```python
from build123d import *

# Parameters (mm, degrees)
SKETCH1_W                                            = 50
SKETCH1_H                                            = 68
BOSS_EXTRUDE1_DEPTH                                  = 8
M3_CLEARANCE_HOLE1_D                                 = 3.4
CSK_FOR_M4_HEX_SOCKET_COUNTERSUNK_CAP_SC_D           = 4.5
CSK_FOR_M4_HEX_SOCKET_COUNTERSUNK_CAP_SC_CSINK_D     = 8.96
CSK_FOR_M4_HEX_SOCKET_COUNTERSUNK_CAP_SC_CSINK_ANGLE = 90
FILLET1_R                                            = 2
CSK_FOR_M4_HEX_SOCKET_COUNTERSUNK_CA_2_D             = 4.5
CSK_FOR_M4_HEX_SOCKET_COUNTERSUNK_CA_2_CSINK_D       = 8.96
CSK_FOR_M4_HEX_SOCKET_COUNTERSUNK_CA_2_CSINK_ANGLE   = 90


with BuildPart() as part:
    # Sketch1 → Boss-Extrude1 (new body)
    with BuildSketch(Plane(origin=(0, 0, 0), x_dir=(0, 0, -1), z_dir=(1, 0, 0))):
        Rectangle(SKETCH1_W, SKETCH1_H)
    extrude(amount=BOSS_EXTRUDE1_DEPTH)

    # M3 Clearance Hole1 (through all)
    with Locations(Plane(origin=(8, 0, 0), x_dir=(0, 0, -1), z_dir=(1, 0, 0))):
        with Locations((-10, 21), (10, 21), (10, 1), (-10, 1)):
            Hole(M3_CLEARANCE_HOLE1_D / 2)

    # CSK for M4 Hex Socket Countersunk Cap Sc (through all)
    with Locations(Plane.ZY):
        with Locations((-20, -29), (20, -29)):
            CounterSinkHole(CSK_FOR_M4_HEX_SOCKET_COUNTERSUNK_CAP_SC_D / 2, CSK_FOR_M4_HEX_SOCKET_COUNTERSUNK_CAP_SC_CSINK_D / 2, counter_sink_angle=CSK_FOR_M4_HEX_SOCKET_COUNTERSUNK_CAP_SC_CSINK_ANGLE)

    # Fillet1
    fillet1_edges = [part.edges().sort_by_distance(p)[0] for p in [
        (4, -34, -25),
        (4, -34, 25),
        (4, 34, 25),
        (4, 34, -25),
    ]]
    fillet(fillet1_edges, radius=FILLET1_R)

    # CSK for M4 Hex Socket Countersunk Ca 2 (through all)
    with Locations(Plane.ZY):
        with Locations((20, -19), (20, 18.5), (-20, 18.5), (-20, -19)):
            CounterSinkHole(CSK_FOR_M4_HEX_SOCKET_COUNTERSUNK_CA_2_D / 2, CSK_FOR_M4_HEX_SOCKET_COUNTERSUNK_CA_2_CSINK_D / 2, counter_sink_angle=CSK_FOR_M4_HEX_SOCKET_COUNTERSUNK_CA_2_CSINK_ANGLE)


solid = part.part
```
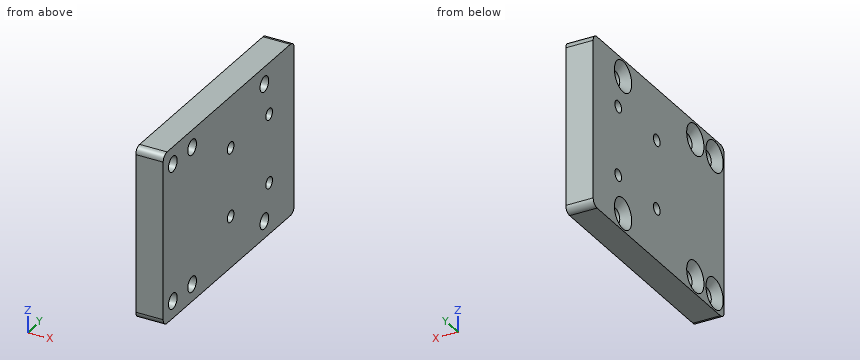
The listing builds one solid part. Answer for the finished solid, in the listing's coordinates (mm). Coordinates: 2 decimals unless noted, no trailing zeros. Write each loop counter-clockwise with the first axis right and the second up, starting at its lowest first coordinate (ties: lowest second). Pieces come first, ordered by that corner, then holes. Notation, with made-up numbers: (68, 29) - (74, 29) arc R34 ccw to (74, 66) - close; hole circle Ø2 at (-21, 48). An arc over 180 degrees is marked (long way). One line per item, written item: value.
1) Find section C-C (y = 1). Give the vertices of the cut face in (x, z).
Geometry check:
outline: (0, -25) - (8, -25) - (8, -11.7) - (0, -11.7) - close; (0, -8.3) - (8, -8.3) - (8, 8.3) - (0, 8.3) - close; (0, 11.7) - (8, 11.7) - (8, 25) - (0, 25) - close
2) Each of these flat-tipped pins is pushed along its axis until it touches: pin 1 Ø5 at (y, z) = (-19, -20) entering from -X; pin 2 Ø2 at (y, z) = (22, -3) entering from -X; pin 3 Ø6 at (y, z) = (18.5, 20) entering from -X. Where does it stop, or does it pass through?
Geometry check:
pin 1: stops at x = 1.98
pin 2: stops at x = 0
pin 3: stops at x = 1.48
3) Find section A-A (z = 10). Give the vertices of the cut face in (x, y), and give its area (3 significant figures).
Geometry check:
outline: (0, -34) - (8, -34) - (8, -0.7) - (0, -0.7) - close; (0, 2.7) - (8, 2.7) - (8, 19.3) - (0, 19.3) - close; (0, 22.7) - (8, 22.7) - (8, 34) - (0, 34) - close
area: 490 mm2
4) Find section B-B (x = 3). Count the separate pieces of the cut face and the enclosed holes in it, and give its area (3 significant figures).
Geometry check:
separate pieces: 1
enclosed holes: 10
area: 3,260 mm2
5) Consider line 1 along Y through (x, z) = (3.55, 20); line 2 along Z through (x, y) = (6.35, -29); line 3 along Y through (x, z) = (6, 10). Determine where each line is inside the solid, lowest interval first. Write a range as from..to.
Geometry check:
line 1: y = -34..-31.25, -26.75..-21.25, -16.75..16.25, 20.75..34
line 2: z = -25..-22.25, -17.75..17.75, 22.25..25
line 3: y = -34..-0.7, 2.7..19.3, 22.7..34
6) Find section D-D (z = -20). Give the vertices of the cut face in (x, y).
Geometry check:
outline: (0, -34) - (8, -34) - (8, -31.25) - (2.23, -31.25) - (0, -33.48) - close; (0, -24.52) - (2.23, -26.75) - (8, -26.75) - (8, -21.25) - (2.23, -21.25) - (0, -23.48) - close; (0, -14.52) - (2.23, -16.75) - (8, -16.75) - (8, 16.25) - (2.23, 16.25) - (0, 14.02) - close; (0, 22.98) - (2.23, 20.75) - (8, 20.75) - (8, 34) - (0, 34) - close
